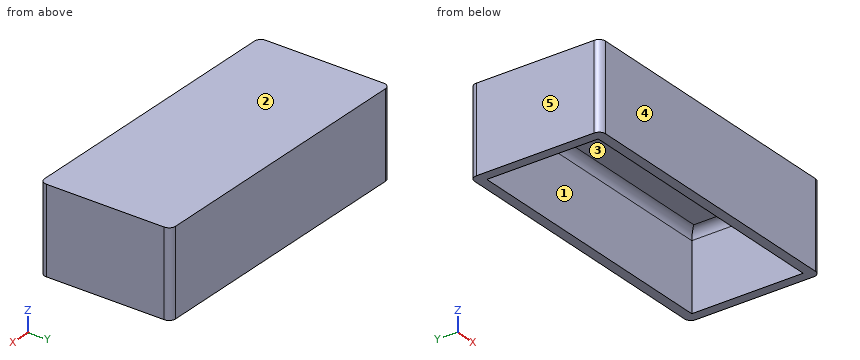
```python
from build123d import *

# Parameters (mm, degrees)
F0_W     = 1800
F0_H     = 800
F1_DEPTH = 520
F2_T     = -60
F3_R     = 50
F4_R     = 40


with BuildPart() as f1:
    # F0 (on Top) → F1 (new body)
    with BuildSketch(Plane.XY):
        Rectangle(F0_W, F0_H)
    extrude(amount=F1_DEPTH)

    # F2
    f2_openings = [f1.faces().sort_by_distance(p)[0] for p in [
        (0, 0, 0),
    ]]
    offset(amount=F2_T, openings=f2_openings)

    # F3
    f3_edges = [f1.edges().sort_by_distance(p)[0] for p in [
        (0, -340, 460),
        (840, 0, 460),
        (0, 340, 460),
        (-840, 0, 460),
    ]]
    fillet(f3_edges, radius=F3_R)

    # F4
    f4_edges = [f1.edges().sort_by_distance(p)[0] for p in [
        (900, 400, 260),
        (900, -400, 260),
        (-900, -400, 260),
        (-900, 400, 260),
    ]]
    fillet(f4_edges, radius=F4_R)


solid = f1.part
```
Source: CAD feature listing. Evaluate the final solid. Frame: model axes, mm. Face numbers are marked on the shaded views. A direction names the side the tool comes from. Round coordinates to 2 decimals unless told otherwise and drop trailing zeros. Loops run counter-clockwise (first coordinate to the right, second up) from the corner with the lowest first, then second, coordinate; pieces in that order, holes last.
(1) Pull-direction query (Y, two-part tool) for the marked faces 3, 4 and 5; classes: +Y half, -Y half, draft (parallel to the pull), parting line (faces both ways), or undercut.
From the geometry:
face 3: undercut
face 4: -Y half
face 5: draft
(2) Material intervals for probe 1 along Y at (x, z) = (206, 173.5); probe 2 along X at (y, z) = (51, 333); probe 3 along X at (y, z) = (-130.5, 414), sorted ascending.
From the geometry:
probe 1: y = -400 to -340, 340 to 400
probe 2: x = -900 to -840, 840 to 900
probe 3: x = -900 to -839.84, 839.84 to 900
(3) Section query A-A (z = 219.5). Output: boundary loops of the cut face in (x, y).
From the geometry:
outline: (-900, -360) arc R40 ccw to (-860, -400) - (860, -400) arc R40 ccw to (900, -360) - (900, 360) arc R40 ccw to (860, 400) - (-860, 400) arc R40 ccw to (-900, 360) - close; hole (-840, -340) - (840, -340) - (840, 340) - (-840, 340) - close
(4) Section query B-B (y = -10). Output: boundary loops of the cut face in (x, z).
From the geometry:
outline: (-900, 0) - (-840, 0) - (-840, 410) arc R50 cw to (-790, 460) - (790, 460) arc R50 cw to (840, 410) - (840, 0) - (900, 0) - (900, 520) - (-900, 520) - close
(5) Access query for the marked faces 1 and 2. Directions: +Z, -Z, +X, -X, +Y, -Y. A direction counts if a zero-diameter tool reaches every point of the face in a straight line with its end or side. Return the directions, or none.
From the geometry:
face 1: -Z
face 2: +Z, +X, -X, +Y, -Y
(6) Contact query for a flat-ended pin moving along its axis: pin 1 Ø1 at (x, y) = (263.5, 5) entering from -Z. Output: stop coordinate, or through.
From the geometry:
pin 1: stops at z = 460
(7) Section query C-C (x = -597). Output: boundary loops of the cut face in (y, z).
From the geometry:
outline: (-400, 0) - (-340, 0) - (-340, 410) arc R50 cw to (-290, 460) - (290, 460) arc R50 cw to (340, 410) - (340, 0) - (400, 0) - (400, 520) - (-400, 520) - close
